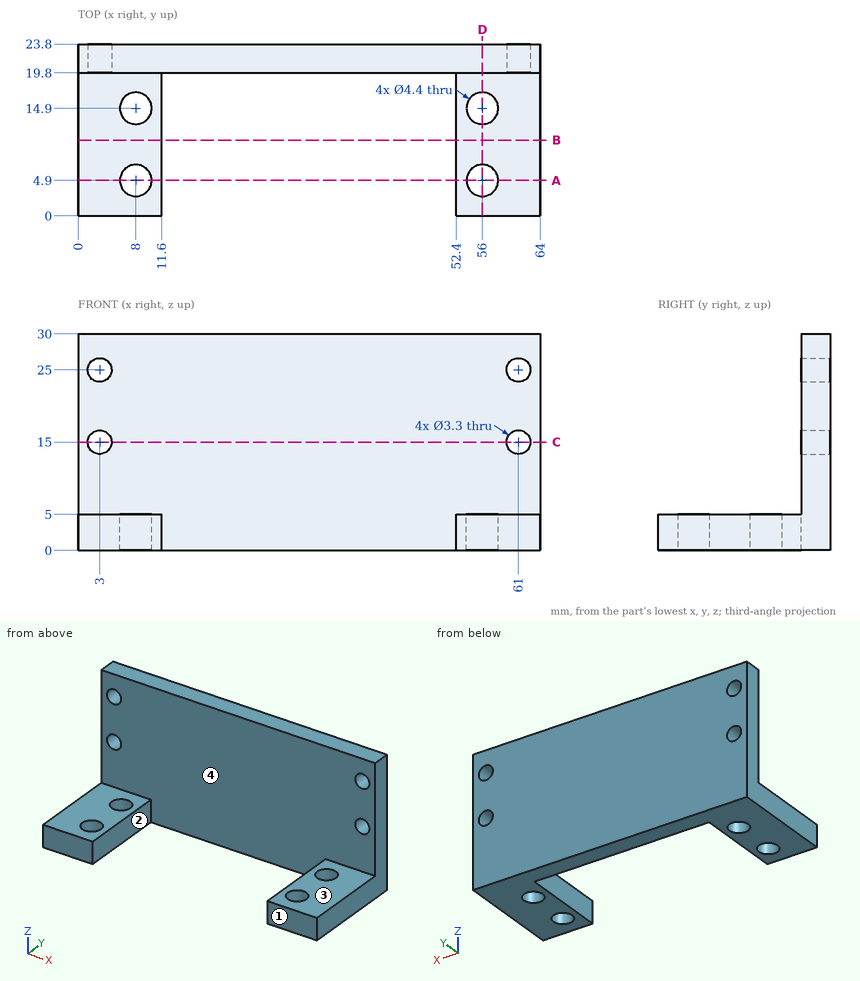
Check sheet for the drawn part. Datum: minimum x, y, z corner. Units: mm. A direction names the side the tool comes from. Coordinates: 2 decimals unless noted, no trailing zeros. Loops run counter-clockwise (first coordinate to the right, second up) from the corner with the lowest first, then second, coordinate; pieces in that order, holes last. Notation, with made-up numbers: (16.25, 69.5) -> (65.25, 69.5) arc R18 cw to (65.25, 104.5) -> close; hole circle Ø9 at (83, 4.25). An arc over 180 degrees is marked (long way). Answer as a JSON object with one key per item and string values. Group by question number.
Item 1: Sectioned sample at C-C on z = 15. Record the boundary of the cut face in (x, y), plus the area to 3 significant figures.
Item 2: Scan lines: probe 1 along Z at (x, y) = (61, 20.85); probe 2 along X at (y, z) = (22.5, 25); probe 3 along Y at (x, z) = (8, 3.2). Record each from-to range of solid material in increasing order.
Item 3: Sectioned sample at D-D on x = 56. Record the boundary of the cut face in (y, z).
Item 4: Depth check by flat-ended pin: pin 1 (10 mm diameter, centred on x = 44.5, z = 20.5, fed in from -Y); pin 2 (12 mm diameter, centred on y = 2.5, z = 15, fed in from +X); pin 3 (9.5 mm diameter, centred on x = 58.5, y = 12, fed in from +Z). Enter the tip coordinate at first touch or a pass-through.
Item 5: Sectioned sample at B-B on y = 10.5. Record the boundary of the cut face in (x, z).
Item 6: Sectioned sample at A-A on y = 4.9. Record the boundary of the cut face in (x, z), plus the area to 3 significant figures.
Item 7: Tool access check on the marked faces 1, 2, 3 and 4. Record the directions out of +Z, -Z, +X, -X, +Y, -Y that give a thin tool (end or side, any length) a straight path to the whole face; none if there is none.
Evaluation:
{
 "1": {"outline": "(0, 19.8) -> (1.35, 19.8) -> (1.35, 23.8) -> (0, 23.8) -> close; (4.65, 19.8) -> (59.35, 19.8) -> (59.35, 23.8) -> (4.65, 23.8) -> close; (62.65, 19.8) -> (64, 19.8) -> (64, 23.8) -> (62.65, 23.8) -> close", "area": "230 mm²"},
 "2": {"probe 1": "z = 0 to 13.35, 16.65 to 23.35, 26.65 to 30", "probe 2": "x = 0 to 1.35, 4.65 to 59.35, 62.65 to 64", "probe 3": "y = 0 to 2.7, 7.1 to 12.7, 17.1 to 23.8"},
 "3": {"outline": "(0, 0) -> (2.7, 0) -> (2.7, 5) -> (0, 5) -> close; (7.1, 0) -> (12.7, 0) -> (12.7, 5) -> (7.1, 5) -> close; (17.1, 0) -> (23.8, 0) -> (23.8, 30) -> (19.8, 30) -> (19.8, 5) -> (17.1, 5) -> close"},
 "4": {"pin 1": "stops at y = 19.8", "pin 2": "passes through", "pin 3": "stops at z = 5"},
 "5": {"outline": "(0, 0) -> (11.6, 0) -> (11.6, 5) -> (0, 5) -> close; (52.4, 0) -> (64, 0) -> (64, 5) -> (52.4, 5) -> close"},
 "6": {"outline": "(0, 0) -> (5.8, 0) -> (5.8, 5) -> (0, 5) -> close; (10.2, 0) -> (11.6, 0) -> (11.6, 5) -> (10.2, 5) -> close; (52.4, 0) -> (53.8, 0) -> (53.8, 5) -> (52.4, 5) -> close; (58.2, 0) -> (64, 0) -> (64, 5) -> (58.2, 5) -> close", "area": "72.0 mm²"},
 "7": {"face 1": "+Z, -Z, +X, -X, -Y", "face 2": "+Z, -Z, -Y", "face 3": "+Z, +X, -X, -Y", "face 4": "+Z, -Y"}
}
